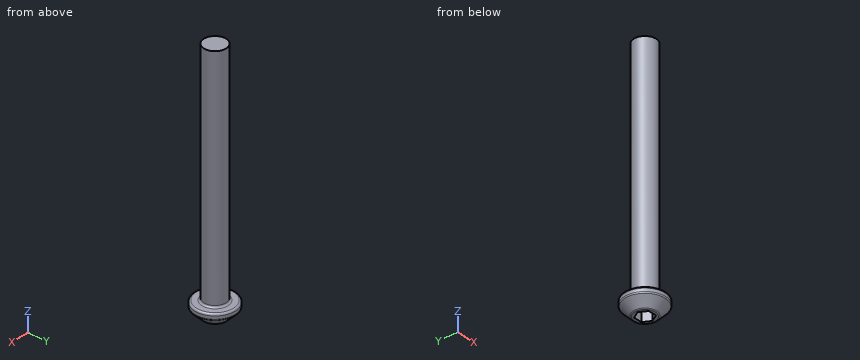
from build123d import *

# Parameters (mm, degrees)
F1_R     = 2.75
F1_R_2   = 1.5
F2_DEPTH = 2
F3_START = 1.5
F3_DEPTH = 0.5
F4_START = 2
F4_DEPTH = 31
F5_SIZE2 = 1.25
F5_SIZE  = 1.25
F6_R     = 0.25


# Not quite as in the source:
# - a feature names something its author has since deleted; it is built from what else it names


with BuildPart() as f2:
    # F1 (on Top) → F2 (new body)
    with BuildSketch(Plane.XY):
        Circle(F1_R)
        Circle(F1_R_2, mode=Mode.SUBTRACT)
        Circle(F1_R_2)
        Polygon((-0.5773502692, -1), (-1.1547005384, 0), (-0.5773502692, 1), (0.5773502692, 1), (1.1547005384, 0), (0.5773502692, -1), align=None, mode=Mode.SUBTRACT)
    extrude(amount=F2_DEPTH)

    # F1 (on Top) → F3 (join)
    with BuildSketch(Plane.XY.offset(F3_START)):
        Polygon((-0.5773502692, 1), (-1.1547005384, 0), (-0.5773502692, -1), (0.5773502692, -1), (1.1547005384, 0), (0.5773502692, 1), align=None)
    extrude(amount=F3_DEPTH)

    # F1 (on Top) → F4 (join)
    with BuildSketch(Plane.XY.offset(F4_START)):
        Circle(F1_R_2)
        Polygon((-0.5773502692, -1), (-1.1547005384, 0), (-0.5773502692, 1), (0.5773502692, 1), (1.1547005384, 0), (0.5773502692, -1), align=None, mode=Mode.SUBTRACT)
        Polygon((-0.5773502692, 1), (-1.1547005384, 0), (-0.5773502692, -1), (0.5773502692, -1), (1.1547005384, 0), (0.5773502692, 1), align=None)
    extrude(amount=F4_DEPTH)

    # F5
    f5_edges = [f2.edges().sort_by_distance(p)[0] for p in [
        (-2.75, 0, 0),
    ]]
    chamfer(f5_edges, length=F5_SIZE, length2=F5_SIZE2)

    # F6
    f6_edges = [f2.edges().sort_by_distance(p)[0] for p in [
        (-2.75, 0, 2),
        (-1.5, 0, 2),
        (-1.5, 0, 0),
        (-2.75, 0, 1.25),
    ]]
    fillet(f6_edges, radius=F6_R)


solid = f2.part
Verification items for the finished model (mm, model axes). Coordinates: 2 decimals unless noted, no trailing zeros. Write each loop counter-clockwise with the first axis right and the second up, starting at its lowest first coordinate (ties: lowest second). Pieces come first, ordered by that corner, then holes. Notation, with made-up numbers: (-28, 59) - (-13, 59) arc R32 cw to (-13, 92) - close; hole circle Ø5 at (85, 14). An arc over 180 degrees is marked (long way). Answer as a JSON object with one key per item and string values.
(1) Gauge pin test, flat ends, axial feed: pin 1 Ø0.6 at (x, z) = (0, 1) entering from -Y; pin 2 Ø1 at (x, z) = (1, 13.5) entering from -Y. Record the tip position at first contact, or that the pin passes through.
Report:
{"pin 1": "y = -2.74", "pin 2": "y = -1.41"}
(2) Thickness scan on line 1 along Z through (x, y) = (-0.55, 0.4); line 2 along Y through (x, z) = (0.05, 14); line 3 along Y through (x, z) = (1.35, 31.5). Record the ranges inside material, lowest first.
Report:
{"line 1": "1.5 to 33", "line 2": "-1.5 to 1.5", "line 3": "-0.65 to 0.65"}
(3) Cross-section at A-A on z = 28. Record the cut outline in (x, y), plus the area to 3 significant figures.
Report:
{"outline": "circle Ø3 at (0, 0)", "area": "7.07 mm^2"}
